```python
from build123d import *

# Parameters (mm, degrees)
F1_DEPTH = 50.8
F2_R     = 12.7
F3_DEPTH = 50.8
F4_W     = 25.4
F4_H     = 25.4
F5_DEPTH = 12.7
F6_R     = 11.122921
F7_DEPTH = 12.7


with BuildPart() as f1:
    # F0 (on Front) → F1 (new body)
    with BuildSketch(Plane.XZ):
        Polygon((-25.4, 0), (0, 0), (25.4, 0), (25.4, 50.8), (-25.4, 50.8), align=None)
    extrude(amount=F1_DEPTH)

    # F2 (on face) → F3 (cut)
    with BuildSketch(Plane.XZ.offset(50.8)):
        with Locations((0, 24.496891)):
            Circle(F2_R)
    extrude(amount=-F3_DEPTH, mode=Mode.SUBTRACT)

    # F4 (on face) → F5 (join)
    with BuildSketch(Plane(origin=(0, 0, 0), x_dir=(1, 0, 0), z_dir=(0, 0, -1))):
        with Locations((-0.931334, 26.528889)):
            Rectangle(F4_W, F4_H)
    extrude(amount=F5_DEPTH)

    # F6 (on face) → F7 (join)
    with BuildSketch(Plane(origin=(-25.4, 0, 0), x_dir=(0, -1, 0), z_dir=(-1, 0, 0))):
        with Locations((25.089554, 27.065113)):
            Circle(F6_R)
    extrude(amount=F7_DEPTH)


solid = f1.part
```
Source: CAD feature listing. Evaluate the final solid. Frame: model axes, mm. A direction names the side the tool comes from. Coordinates: 2 decimals unless noted, no trailing zeros. Order: outer loops, then holes, each group sorted by start corner. A loop starts at its lowest first (then second) coordinate and runs counter-clockwise, first axis right, second up. Notation, with made-up numbers: M -26.5,51.5 L 16.5,51.5 A17 ccw 16.5,70.5 Z; hole C 63,-25.5 d11. An arc over 180 degrees is marked long. Write each question's results on one line, items separated by ' | '. Start each with the question number.
1) Section query D-D (x = 18.5). Return the cut outline in (y, z), plus the area to 3 significant figures.
2) Section query C-C (y = -33.5). Return the cut outline in (x, z), plus the area to 3 significant figures.
3) Access query for faces 1 (the face through (-31.7, -35.7, 30.4)), 2 (the face through (-13.631, -26, -6)), 3 (the face through (-1, -39.229, -6)). Directions: +Z, -Z, +X, -X, +Y, -Y. A direction counts if a zero-diameter tool reaches every point of the face in a straight line with its end or side. Return the directions, or none.
4) Section query A-A (x = 0). Return the cut outline in (y, z), plus the area to 3 significant figures.
5) Draft query along X for faces 4 (the face through (11.769, -26, -6)), 5 (the face through (-1.65, -25.76, 37.09)), 6 (the face through (-1, -13.829, -6)). Return one class per face: released by +X, released by -X, zero draft, split by the parting line, or undercut.
6) Line query: line 1 (Z direction, x = 0, y = -15); line 2 (Z direction, x = -15.5, y = -27.5); line 3 (X direction, y = -4, z = 28). Output: solid intervals per line, ascending. Write a range as from..to.
7) Contact query for flat-ended pins moving along their axis: pin 1 Ø6 at (y, z) = (-10, -3.5) entering from -X; pin 2 Ø5 at (x, y) = (3, -8) entering from -Z; pin 3 Ø10 at (y, z) = (-22, -9) entering from -X; pin 4 Ø4 at (y, z) = (-30, -9) entering from +X. Output: stop coordinate, or through.
8) Section query B-B (z = 31.5). Return the cut outline in (x, y).
Answers:
1) outline: M -50.8,0 L 0,0 L 0,50.8 L -50.8,50.8 Z | area: 2,580 mm^2
2) outline: M -38.1,19.79 L -25.4,19.79 L -25.4,0 L -13.63,0 L -13.63,-12.7 L 11.77,-12.7 L 11.77,0 L 25.4,0 L 25.4,50.8 L -25.4,50.8 L -25.4,34.34 L -38.1,34.34 Z; hole C 0,24.5 d25.4 | area: 2,580 mm^2
3) face 1: -X | face 2: -Z, -X, +Y, -Y | face 3: -Z, +X, -X, -Y
4) outline: M -50.8,0 L -39.23,0 L -39.23,-12.7 L -13.83,-12.7 L -13.83,0 L 0,0 L 0,11.8 L -50.8,11.8 Z; M -50.8,37.2 L 0,37.2 L 0,50.8 L -50.8,50.8 Z | area: 1,610 mm^2
5) face 4: released by +X | face 5: undercut | face 6: zero draft
6) line 1: z = -12.7..11.8, 37.2..50.8 | line 2: z = 0..50.8 | line 3: x = -25.4..-12.21, 12.21..25.4
7) pin 1: passes through | pin 2: stops at z = 0 | pin 3: stops at x = -13.63 | pin 4: stops at x = 11.77
8) outline: M -38.1,-35.29 L -25.4,-35.29 L -25.4,-50.8 L -10.59,-50.8 L -10.59,0 L -25.4,0 L -25.4,-14.89 L -38.1,-14.89 Z; M 10.59,-50.8 L 25.4,-50.8 L 25.4,0 L 10.59,0 Z
